Can you work these out from the model? Positions are in its coordinate system, mm. A direction names the side the tool comes from. Round coordinates to 2 decimals unless told otherwise and drop trailing zeros. Order: outer loops, then holes, each group sorted by start corner. A loop starts at its lowest first (then second) coordinate and runs counter-clockwise, first axis right, second up.
Q1. If we section it at D-D (x = 2.5): Please give me the cut outline in (y, z).
Q2. If we section it at B-B (z = -1.75): Please give me the cut outline in (x, y).
Q3. For faces 3 (the face through (4.8, -1, 0)), 4 (the face through (7, -3, 0)), 5 (the face through (3, 0, 2)), which set-ups out of +Z, -Z, +X, -X, +Y, -Y let a thin tool reach every point of the face, with its end or its side?
Q4. If we section it at A-A (x = 0): Please give me the cut outline in (y, z).
Q5. If I drill on line 1 (X direction, y = 0.1, z = 0); line 2 (Y direction, x = 6.5, z = -0.5); line 3 (X direction, y = -2.35, z = 0.75), over which ranges is the centre line in solid material (lowest first)?
Q6. Will these pins go through, and if not, where does the flat tip stop? P1, Ø4, axis at x = 1, z = 1.5, coming from the -Y side; P2, Ø1.9, axis at x = 4.5, y = -0.5, coming from the -Z side; P3, Ø0.7, axis at x = 5, y = -1, coming from the +Z side.
Q7. If we section it at C-C (y = -1): Please give me the cut outline in (x, z).
Q8. We'd pull the mould along Z, two halves only. Please class faces 1 (the face through (3.42, 0.15, -0.45)), 2 (the face through (3, 0.3, -2)): pulls with the +Z half, pulls with the -Z half, needs draft (parallel to the pull), parting line crosses it, or undercut.
from build123d import *

# Parameters (mm, degrees)
SKETCH_1_R          = 3.45
EXTRUDE_1_DEPTH     = 0.3
SKETCH_2_W          = 8.378641338
SKETCH_2_H          = 6.913843901
CUT_EXTRUDE_1_DEPTH = 10
EXTRUDE_2_DEPTH     = 3.8
FILLET_1_R          = 1.9
CUT_EXTRUDE_2_DEPTH = 10


with BuildPart() as part:
    # 草图1 → 凸台-拉伸1 (new body)
    with BuildSketch(Plane(origin=(0, 0, 0), x_dir=(1, 0, 0), z_dir=(0, 1, 0))):
        with BuildLine():
            Line((3.519943181, 1.9), (10, 1.9))
            ThreePointArc((10, 1.9), (11.9, 0), (10, -1.9))
            Line((10, -1.9), (3.519943181, -1.9))
            ThreePointArc((3.519943181, -1.9), (-4, 0), (3.519943181, 1.9))
        make_face()
        with Locations(Location((0, 0, 0), (0, 0, 270))):
            Circle(SKETCH_1_R, mode=Mode.SUBTRACT)
        with BuildLine():
            Line((10, -0.6), (8.5, -0.6))
            ThreePointArc((8.5, -0.6), (7.9, 0), (8.5, 0.6))
            Line((8.5, 0.6), (10, 0.6))
            ThreePointArc((10, 0.6), (10.6, 0), (10, -0.6))
        make_face(mode=Mode.SUBTRACT)
    extrude(amount=EXTRUDE_1_DEPTH)

    # 草图2 → 切除-拉伸1 (cut)
    with BuildSketch(Plane(origin=(0, 0.3, 0), x_dir=(1, 0, 0), z_dir=(0, 1, 0))):
        with Locations((8.689320669, -0.04590274)):
            Rectangle(SKETCH_2_W, SKETCH_2_H)
    extrude(amount=-CUT_EXTRUDE_1_DEPTH, mode=Mode.SUBTRACT)

    # 草图3 → 凸台-拉伸2 (add)
    with BuildSketch(Plane.XY.offset(1.9)):
        Polygon((4.5, 0.3), (4.8, 0.3), (4.8, -2.7), (7.8, -2.7), (7.8, -3), (4.5, -3), (4.5, 0), align=None)
    extrude(amount=-EXTRUDE_2_DEPTH)

    # 圆角1
    fillet_1_edges = [part.edges().sort_by_distance(p)[0] for p in [
        (7.8, -2.85, -1.9),
        (7.8, -2.85, 1.9),
    ]]
    fillet(fillet_1_edges, radius=FILLET_1_R - 0.0001)  # a hair under: the kernel refuses the full size

    # 草图4 → 切除-拉伸2 (cut)
    with BuildSketch(Plane(origin=(0, -2.7, 0), x_dir=(1, 0, 0), z_dir=(0, 1, 0))):
        with BuildLine():
            Line((5.9, -0.6), (4.4, -0.6))
            ThreePointArc((4.4, -0.6), (3.8, 0), (4.4, 0.6))
            Line((4.4, 0.6), (5.9, 0.6))
            ThreePointArc((5.9, 0.6), (6.5, 0), (5.9, -0.6))
        make_face()
    extrude(amount=-CUT_EXTRUDE_2_DEPTH, mode=Mode.SUBTRACT)


solid = part.part
Solution:
1. outline: (0, -3.12) - (0.3, -3.12) - (0.3, -2.38) - (0, -2.38) - close; (0, 2.38) - (0.3, 2.38) - (0.3, 3.12) - (0, 3.12) - close
2. outline: (-3.6, 0) - (-2.97, 0) - (-2.97, 0.3) - (-3.6, 0.3) - close; (2.97, 0) - (4.5, 0) - (4.5, -3) - (6.64, -3) - (6.64, -2.7) - (4.8, -2.7) - (4.8, 0.3) - (2.97, 0.3) - close
3. face 3: +Z, -Z, +X, +Y
3. face 4: +Z, -Z, +X, -X, -Y
3. face 5: +Z, -Z, -X, -Y
4. outline: (0, -4) - (0.3, -4) - (0.3, -3.45) - (0, -3.45) - close; (0, 3.45) - (0.3, 3.45) - (0.3, 4) - (0, 4) - close
5. line 1: x = -4 to -3.45, 3.45 to 4.8
5. line 2: y = -3 to -2.7
5. line 3: x = 4.5 to 4.8
6. P1: stops at y = 0
6. P2: stops at z = -1.9
6. P3: stops at z = 1.9
7. outline: (4.5, -1.9) - (4.8, -1.9) - (4.8, 1.9) - (4.5, 1.9) - close
8. face 1: undercut
8. face 2: needs draft
